Geometry: final body of the model. Coordinates: model frame, mm. A direction names the side the tool comes from. Give positions to 0.01 mm unless a question says otherwise; leave off trailing zeros. Write each loop counter-clockwise with the first axis right and the second up, starting at its lowest first coordinate (ties: lowest second). Pieces come first, ordered by that corner, then holes. Notation, with made-up numbers: (-14, -27) -> (22, -27) arc R19 ccw to (22, -6) -> close; hole circle Ø9 at (58.5, 33). An arc over 180 degrees is marked (long way). Answer in a Markdown table with one row per item. Add a question column.
Item 1: Access query for faces 4 (the flat face through (-2, -35, 150)), 5 (the flat face through (-2, -35, -144)). Directions: +Z, -Z, +X, -X, +Y, -Y. A direction counts if a zero-diameter tool reaches every point of the face in a straight line with its end or side. Return the directions, or none.
Item 2: Section query C-C on z = -12.5. Output: boundary loops of the cut face in (x, y), plus the area to 3 significant figures.
Item 3: Draft query along X for faces 1 (the cylindrical face through (-236.49, -34.51, -109.72)), 2 (the flat face through (-2, -35, -150)), 3 (the cylindrical face through (238.915, -34.51, 115.781)). Return one class per face: +X half, -X half, draft (parallel to the pull), parting line (faces both ways), or undercut.
Item 4: Section query B-B on x = 107.5. Output: boundary loops of the cut face in (y, z).
Item 5: First-contact query: P1, Ø3, axis at y = -118, z = 119, coming from the +X side; P2, Ø12, axis at x = 149, z = -107.5, coming from the -Y side; P3, Ø1.5, axis at x = -163.5, z = 19, coming from the +Y side. Flat tips, straight axial feed; report the tip coordinate or a pass-through.
Item 6: Section query A-A on y = -43.5. Output: boundary loops of the cut face in (x, z), plus the area to 3 significant figures.
Item 7: Material intervals for probe 1 along Z at (x, y) = (-154, -66); probe 2 along Y at (x, z) = (-50, -11.5); probe 3 along X at (y, z) = (-36, 52.5), sorted ascending. Write a range as from..to.
```python
from build123d import *

# Parameters (mm, degrees)
CROQUIS1_W              = 550
CROQUIS1_H              = 150
SALIENTE_EXTRUIR1_DEPTH = 150
REDONDEO1_R             = 120
REDONDEO2_R             = 80
VACIADO1_T              = -6


with BuildPart() as part:
    # Croquis1 → Saliente-Extruir1 (new body, symmetric)
    with BuildSketch(Plane.XY):
        with Locations((0, -75)):
            Rectangle(CROQUIS1_W, CROQUIS1_H)
    extrude(amount=SALIENTE_EXTRUIR1_DEPTH, both=True)

    # Redondeo1
    redondeo1_edges = [part.edges().sort_by_distance(p)[0] for p in [
        (275, -75, 150),
        (-275, -75, 150),
        (275, -75, -150),
        (-275, -75, -150),
    ]]
    fillet(redondeo1_edges, radius=REDONDEO1_R)

    # Redondeo2
    redondeo2_edges = [part.edges().sort_by_distance(p)[0] for p in [
        (275, -150, 0),
        (0, -150, -150),
        (0, -150, 150),
        (-275, -150, 0),
        (-239.852813742, -150, 114.852813742),
        (-239.852813742, -150, -114.852813742),
        (239.852813742, -150, 114.852813742),
        (239.852813742, -150, -114.852813742),
    ]]
    fillet(redondeo2_edges, radius=REDONDEO2_R)

    # Vaciado1
    vaciado1_openings = [part.faces().sort_by_distance(p)[0] for p in [
        (0, 0, 0),
    ]]
    offset(amount=VACIADO1_T, openings=vaciado1_openings, kind=Kind.INTERSECTION)


solid = part.part
```
Findings below:
| question | item | result |
|---|---|---|
| 1 | face 4 | +Z, +X, -X, +Y, -Y |
| 1 | face 5 | +Y |
| 2 | outline | (-275, -70) arc R80 ccw to (-195, -150) -> (195, -150) arc R80 ccw to (275, -70) -> (275, 0) -> (269, 0) -> (269, -70) arc R74 cw to (195, -144) -> (-195, -144) arc R74 cw to (-269, -70) -> (-269, 0) -> (-275, 0) -> close |
| 2 | area | 4,630 mm^2 |
| 3 | face 1 | undercut |
| 3 | face 2 | draft |
| 3 | face 3 | +X half |
| 4 | outline | (-150, -70) arc R80 ccw to (-70, -150) -> (0, -150) -> (0, -144) -> (-70, -144) arc R74 cw to (-144, -70) -> (-144, 70) arc R74 cw to (-70, 144) -> (0, 144) -> (0, 150) -> (-70, 150) arc R80 ccw to (-150, 70) -> close |
| 5 | P1 | stops at x = 211.98 |
| 5 | P2 | stops at y = -143.54 |
| 5 | P3 | stops at y = -144 |
| 6 | outline | (-275, -30) arc R120 ccw to (-155, -150) -> (155, -150) arc R120 ccw to (275, -30) -> (275, 30) arc R120 ccw to (155, 150) -> (-155, 150) arc R120 ccw to (-275, 30) -> close; hole (-269, -30) arc R114 ccw to (-155, -144) -> (155, -144) arc R114 ccw to (269, -30) -> (269, 30) arc R114 ccw to (155, 144) -> (-155, 144) arc R114 ccw to (-269, 30) -> close |
| 6 | area | 8,850 mm^2 |
| 7 | probe 1 | z = -150..-144, 144..150 |
| 7 | probe 2 | y = -150..-144 |
| 7 | probe 3 | x = -272.87..-266.76, 266.76..272.87 |
